```python
from build123d import *

# Parameters (mm, degrees)
SKETCH1_R               = 17
BOSS_EXTRUDE2_DEPTH     = 2.705
BOSS_EXTRUDE3_DEPTH     = 4.39
SKETCH6_3_R             = 6.9
CUT_EXTRUDE2_DEPTH      = 5.39
CUT_EXTRUDE2_DEPTH_BACK = 6.41
SKETCH6_6_R             = 8.14
CUT_EXTRUDE3_DEPTH      = 4.11
SKETCH6_7_R             = 8.14
SKETCH6_7_R_2           = 6.9
CUT_EXTRUDE4_DEPTH      = 2.61
SKETCH6_12_R            = 1.04
SKETCH6_12_R_2          = 1.048997708
CUT_EXTRUDE5_DEPTH      = 6.41
SKETCH6_13_R            = 2.08
SKETCH6_13_R_2          = 1.04
SKETCH6_13_R_3          = 1.048997708
BOSS_EXTRUDE4_DEPTH     = 7.61


with BuildPart() as part:
    # Sketch1 → Boss-Extrude2 (new body, symmetric)
    with BuildSketch(Plane.XY):
        Circle(SKETCH1_R)
    extrude(amount=BOSS_EXTRUDE2_DEPTH, both=True)

    # Sketch6 → Boss-Extrude3 (add)
    with BuildSketch(Plane(origin=(0, 0, -2.705), x_dir=(-1, 0, 0), z_dir=(0, 0, -1))):
        with BuildLine():
            ThreePointArc((-7.785906142, 12.23232053), (0, 14.5), (7.785906142, 12.23232053))
            ThreePointArc((7.785906142, 12.23232053), (8.750658086, 12.703387332), (9.821803695, 12.630604585))
            ThreePointArc((9.821803695, 12.630604585), (0, 16), (-9.821803695, 12.630604585))
            ThreePointArc((-9.821803695, 12.630604585), (-8.750658086, 12.703387332), (-7.785906142, 12.23232053))
        make_face()
        with BuildLine():
            ThreePointArc((10.909063856, 9.552084892), (13.46504185, 5.379837169), (14.487787098, 0.595))
            ThreePointArc((14.487787098, 0.595), (14.5, 0), (14.487787098, -0.595))
            ThreePointArc((14.487787098, -0.595), (13.46504185, -5.379837169), (10.909063856, -9.552084892))
            ThreePointArc((10.909063856, -9.552084892), (11.148155752, -10.084350931), (11.23, -10.662082348))
            ThreePointArc((11.23, -10.662082348), (11.170079442, -11.157742564), (10.993770145, -11.624844859))
            ThreePointArc((10.993770145, -11.624844859), (16, 0), (10.993770145, 11.624844859))
            ThreePointArc((10.993770145, 11.624844859), (11.170079442, 11.157742564), (11.23, 10.662082348))
            ThreePointArc((11.23, 10.662082348), (11.148155752, 10.084350931), (10.909063856, 9.552084892))
        make_face()
        with BuildLine():
            ThreePointArc((9.821803695, -12.630604585), (8.750658086, -12.703387332), (7.785906142, -12.23232053))
            ThreePointArc((7.785906142, -12.23232053), (0, -14.5), (-7.785906142, -12.23232053))
            ThreePointArc((-7.785906142, -12.23232053), (-8.750658086, -12.703387332), (-9.821803695, -12.630604585))
            ThreePointArc((-9.821803695, -12.630604585), (0, -16), (9.821803695, -12.630604585))
        make_face()
        with BuildLine():
            ThreePointArc((-14.487787098, 0.595), (-13.46504185, 5.379837169), (-10.909063856, 9.552084892))
            ThreePointArc((-10.909063856, 9.552084892), (-11.228265305, 10.577151075), (-10.993770145, 11.624844859))
            ThreePointArc((-10.993770145, 11.624844859), (-16, 0), (-10.993770145, -11.624844859))
            ThreePointArc((-10.993770145, -11.624844859), (-11.228265305, -10.577151075), (-10.909063856, -9.552084892))
            ThreePointArc((-10.909063856, -9.552084892), (-13.46504185, -5.379837169), (-14.487787098, -0.595))
            ThreePointArc((-14.487787098, -0.595), (-14.5, 0), (-14.487787098, 0.595))
        make_face()
        with BuildLine():
            Line((-12.1, 0.595), (-14.487787098, 0.595))
            ThreePointArc((-14.487787098, 0.595), (-14.5, 0), (-14.487787098, -0.595))
            Line((-14.487787098, -0.595), (-12.1, -0.595))
            Line((-12.1, -0.595), (-12.1, 0.595))
        make_face()
        with BuildLine():
            ThreePointArc((14.487787098, -0.595), (14.5, 0), (14.487787098, 0.595))
            Line((14.487787098, 0.595), (12.1, 0.595))
            Line((12.1, 0.595), (12.1, -0.595))
            Line((12.1, -0.595), (14.487787098, -0.595))
        make_face()
    extrude(amount=BOSS_EXTRUDE3_DEPTH)

    # Sketch6<3> → Cut-Extrude2 (cut, two sides)
    with BuildSketch(Plane(origin=(0, 0, -2.705), x_dir=(-1, 0, 0), z_dir=(0, 0, -1))) as cut_extrude2_sk:
        Circle(SKETCH6_3_R)
    extrude(amount=CUT_EXTRUDE2_DEPTH, mode=Mode.SUBTRACT)
    extrude(cut_extrude2_sk.sketch, amount=-CUT_EXTRUDE2_DEPTH_BACK, mode=Mode.SUBTRACT)

    # Sketch6<6> → Cut-Extrude3 (cut)
    with BuildSketch(Plane(origin=(0, 0, -2.705), x_dir=(-1, 0, 0), z_dir=(0, 0, -1))):
        with BuildLine():
            Line((12.1, 0.595), (14.487787098, 0.595))
            ThreePointArc((14.487787098, 0.595), (13.46504185, 5.379837169), (10.909063856, 9.552084892))
            ThreePointArc((10.909063856, 9.552084892), (7.795409253, 9.08363884), (7.785906142, 12.23232053))
            ThreePointArc((7.785906142, 12.23232053), (0, 14.5), (-7.785906142, 12.23232053))
            ThreePointArc((-7.785906142, 12.23232053), (-7.257420382, 11.524951045), (-7.07, 10.662082348))
            ThreePointArc((-7.07, 10.662082348), (-8.572268583, 8.663926596), (-10.909063856, 9.552084892))
            ThreePointArc((-10.909063856, 9.552084892), (-13.46504185, 5.379837169), (-14.487787098, 0.595))
            Line((-14.487787098, 0.595), (-12.1, 0.595))
            Line((-12.1, 0.595), (-12.1, -0.595))
            Line((-12.1, -0.595), (-14.487787098, -0.595))
            ThreePointArc((-14.487787098, -0.595), (-13.46504185, -5.379837169), (-10.909063856, -9.552084892))
            ThreePointArc((-10.909063856, -9.552084892), (-8.572268583, -8.663926596), (-7.07, -10.662082348))
            ThreePointArc((-7.07, -10.662082348), (-7.257420382, -11.524951045), (-7.785906142, -12.23232053))
            ThreePointArc((-7.785906142, -12.23232053), (0, -14.5), (7.785906142, -12.23232053))
            ThreePointArc((7.785906142, -12.23232053), (7.795409253, -9.08363884), (10.909063856, -9.552084892))
            ThreePointArc((10.909063856, -9.552084892), (13.46504185, -5.379837169), (14.487787098, -0.595))
            Line((14.487787098, -0.595), (12.1, -0.595))
            Line((12.1, -0.595), (12.1, 0.595))
        make_face()
        Circle(SKETCH6_6_R, mode=Mode.SUBTRACT)
    extrude(amount=-CUT_EXTRUDE3_DEPTH, mode=Mode.SUBTRACT)

    # Sketch6<7> → Cut-Extrude4 (cut)
    with BuildSketch(Plane(origin=(0, 0, -2.705), x_dir=(-1, 0, 0), z_dir=(0, 0, -1))):
        Circle(SKETCH6_7_R)
        Circle(SKETCH6_7_R_2, mode=Mode.SUBTRACT)
    extrude(amount=-CUT_EXTRUDE4_DEPTH, mode=Mode.SUBTRACT)

    # Sketch6<12> → Cut-Extrude5 (cut, through all)
    with BuildSketch(Plane(origin=(0, 0, -2.705), x_dir=(-1, 0, 0), z_dir=(0, 0, -1))):
        with Locations((9.15, -10.662082348)):
            Circle(SKETCH6_12_R)
        with Locations((-9.15, -10.662082348)):
            Circle(SKETCH6_12_R_2)
        with Locations((9.15, 10.662082348)):
            Circle(SKETCH6_12_R)
        with Locations((-9.15, 10.662082348)):
            Circle(SKETCH6_12_R)
    extrude(amount=-CUT_EXTRUDE5_DEPTH, mode=Mode.SUBTRACT)

    # Sketch6<13> → Boss-Extrude4 (add)
    with BuildSketch(Plane(origin=(0, 0, -2.705), x_dir=(-1, 0, 0), z_dir=(0, 0, -1))):
        with Locations((9.15, 10.662082348)):
            Circle(SKETCH6_13_R)
        with Locations((9.15, 10.662082348)):
            Circle(SKETCH6_13_R_2, mode=Mode.SUBTRACT)
        with Locations((9.15, -10.662082348)):
            Circle(SKETCH6_13_R)
        with Locations((9.15, -10.662082348)):
            Circle(SKETCH6_13_R_2, mode=Mode.SUBTRACT)
        with Locations((-9.15, 10.662082348)):
            Circle(SKETCH6_13_R)
        with Locations((-9.15, 10.662082348)):
            Circle(SKETCH6_13_R_2, mode=Mode.SUBTRACT)
        with Locations((-9.15, -10.662082348)):
            Circle(SKETCH6_13_R)
        with Locations((-9.15, -10.662082348)):
            Circle(SKETCH6_13_R_3, mode=Mode.SUBTRACT)
    extrude(amount=BOSS_EXTRUDE4_DEPTH)


solid = part.part
```
CAD build for the part. Positions are in the model's coordinates, mm. A direction names the side the tool comes from. Round coordinates to 2 decimals unless told otherwise and drop trailing zeros. Order: outer loops, then holes, each group sorted by start corner. A loop starts at its lowest first (then second) coordinate and runs counter-clockwise, first axis right, second up. Notation, with made-up numbers: (38, 82.25) - (51, 82.25) arc R9 cw to (51, 95.25) - close; hole circle Ø11 at (60.25, 41.25). An arc over 180 degrees is marked (long way). Answer as CSV lines item,"result". Start each with the question number.
1. Saw through at D-D, the plane z = -4.5. Write the cut outline in (x, y) (3 decimals), and give its area (3 significant figures).
2. Pull direction Y, two halves, no side cores. Call faces 1 (the face through (-0.1, -14.5, -2.8)), 2 (the face through (16, 0, -5)), 3 (the face through (13, -10, -2.705)): +Y half, -Y half, draft (parallel to the pull), parting line (faces both ways), or undercut.
3. Pin check, flat tips, straight feed: pin 1 (1.9 mm diameter, centred on x = 14, z = -2, fed in from -Y); pin 2 (3 mm diameter, centred on y = 12, z = -2.5, fed in from +X); pin 3 (3.5 mm diameter, centred on x = -9.15, y = -10.66, fed in from -Z) (3 decimals); pin 4 (1.1 mm diameter, centred on x = -1, y = -14.5, fed in from -Z) (3 decimals). Stop position of each tip, or through.
4. Saw through at A-A, the plane z = -8.5. Write the cut outline in (x, y).
5. Saw through at C-C, the plane y = 0. Write the cut outline in (x, z) (3 decimals).
6. Drill centre lines: L1, parallel to Y at x = -9.15, z = -7.5; L2, parallel to X at y = 0.5, z = -2.5; L3, parallel to Y at x = -7.5, z = 1. Where is each one in solid material? Low to high. Write a range as [from, to].
7. Tool access for faces 4 (the face through (9, 12, -10.315)), 5 (the face through (-16, 0, -5)), 6 (the face through (-12.1, 0, -3)): list every direction of +Z, -Z, +X, -X, +Y, -Y with a clear straight run to the whole face (end or side of a thin tool).
8. Saw through at B-B, the plane x = 0. Write the cut outline in (y, z) (3 decimals), and give its area (3 significant figures).
Model answer:
1,outline,"(-10.994, -11.625) arc R2.08 ccw to (-9.822, -12.631) arc R16 ccw to (9.822, -12.631) arc R2.08 ccw to (10.994, -11.625) arc R16 ccw to (10.994, 11.625) arc R2.08 ccw to (9.822, 12.631) arc R16 ccw to (-9.822, 12.631) arc R2.08 ccw to (-10.994, 11.625) arc R16 ccw to start; hole (-14.488, -0.595) arc R14.5 ccw to (-10.909, -9.552) arc R2.08 cw (long way) to (-7.786, -12.232) arc R14.5 ccw to (7.786, -12.232) arc R2.08 cw (long way) to (10.909, -9.552) arc R14.5 ccw to (14.488, -0.595) - (12.1, -0.595) - (12.1, 0.595) - (14.488, 0.595) arc R14.5 ccw to (10.909, 9.552) arc R2.08 cw (long way) to (7.786, 12.232) arc R14.5 ccw to (-7.786, 12.232) arc R2.08 cw (long way) to (-10.909, 9.552) arc R14.5 ccw to (-14.488, 0.595) - (-12.1, 0.595) - (-12.1, -0.595) - close; hole circle Ø2.08 at (-9.15, -10.662); hole circle Ø2.08 at (-9.15, 10.662); hole circle Ø2.098 at (9.15, -10.662); hole circle Ø2.08 at (9.15, 10.662)"
1,area,"170 mm²"
2,face 1,"undercut"
2,face 2,"parting line"
2,face 3,"draft"
3,pin 1,"stops at y = -10.89"
3,pin 2,"stops at x = 13.37"
3,pin 3,"stops at z = -10.315"
3,pin 4,"stops at z = -7.095"
4,outline,"circle Ø4.16 at (-9.15, -10.66); circle Ø4.16 at (-9.15, 10.66); circle Ø4.16 at (9.15, -10.66); circle Ø4.16 at (9.15, 10.66); hole circle Ø2.08 at (-9.15, -10.66); hole circle Ø2.08 at (-9.15, 10.66); hole circle Ø2.1 at (9.15, -10.66); hole circle Ø2.08 at (9.15, 10.66)"
5,outline,"(-17, -2.705) - (-16, -2.705) - (-16, -7.095) - (-12.1, -7.095) - (-12.1, 1.405) - (-8.14, 1.405) - (-8.14, -0.095) - (-6.9, -0.095) - (-6.9, 2.705) - (-17, 2.705) - close; (6.9, -0.095) - (8.14, -0.095) - (8.14, 1.405) - (12.1, 1.405) - (12.1, -7.095) - (16, -7.095) - (16, -2.705) - (17, -2.705) - (17, 2.705) - (6.9, 2.705) - close"
6,L1,"y = [-12.74, -11.7], [-9.62, -8.58], [8.58, 9.62], [11.7, 12.74]"
6,L2,"x = [-16.99, -12.1], [12.1, 16.99]"
6,L3,"y = [-15.26, -12.41], [-11.93, -9.4], [-3.16, 3.16], [9.4, 11.93], [12.41, 15.26]"
7,face 4,"-Z, +X, -X, +Y, -Y"
7,face 5,"-Z, -X"
7,face 6,"-Z"
8,outline,"(-17, -2.705) - (-16, -2.705) - (-16, -7.095) - (-14.5, -7.095) - (-14.5, 1.405) - (-8.14, 1.405) - (-8.14, -0.095) - (-6.9, -0.095) - (-6.9, 2.705) - (-17, 2.705) - close; (6.9, -0.095) - (8.14, -0.095) - (8.14, 1.405) - (14.5, 1.405) - (14.5, -7.095) - (16, -7.095) - (16, -2.705) - (17, -2.705) - (17, 2.705) - (6.9, 2.705) - close"
8,area,"63.7 mm²"
